Can you work these out from the model? Positions are in its coordinate system, mm. Face numbers are marked on the shaded views. Coordinates: 2 decimals unless noted, no trailing zeros. Loops run counter-clockwise (first coordinate to the right, second up) from the corner with the lowest first, then second, coordinate; pieces in that order, holes last.
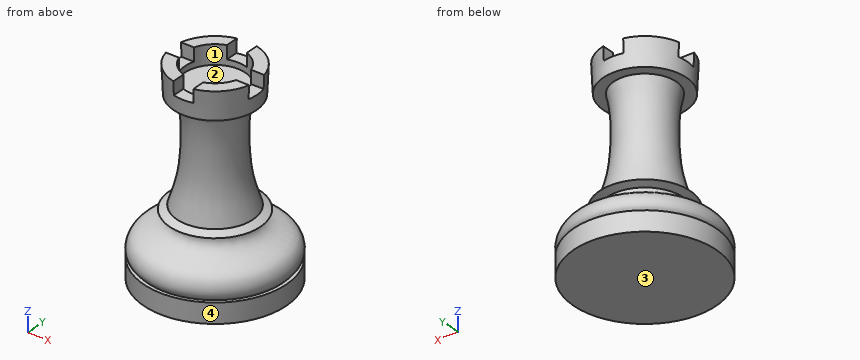
```python
from build123d import *

# Parameters (mm, degrees)
F2_W     = 2.54
F2_H     = 2.54
F3_DEPTH = 1.7018
F4_R     = 3.8696767193
F5_DEPTH = 25.4
F6_DEPTH = 0.762


with BuildPart() as f1:
    # F0 (on Front) → F1 (revolve)
    with BuildSketch(Plane.XZ):
        Polygon((0, 2.54), (0, 0), (9.1186, 0), (9.1186, 2.54), (8.6556235328, 2.54), align=None)
        with BuildLine():
            Line((0, 8.6968354881), (0, 2.54))
            Line((0, 2.54), (8.6556235328, 2.54))
            add(Edge.make_bspline(
                [(8.6556235328, 2.54), (8.8550384762, 2.7402463297), (9.3618805952, 3.2434009078), (8.6917500556, 5.5027157982), (5.7913825103, 5.9282046951), (4.8176161945, 7.0821708068), (4.8696040176, 7.7928476967)],
                knots=[0, 0, 0, 0, 0.1745078988, 0.4312211664, 0.7434636272, 1, 1, 1, 1], degree=3))
            Line((4.8696040176, 7.7928476967), (5.8183851652, 8.18317011))
            Line((5.8183851652, 8.18317011), (4.8696040176, 8.6968354881))
            Line((4.8696040176, 8.6968354881), (0, 8.6968354881))
        make_face()
        with BuildLine():
            Line((0, 25.4), (0, 8.6968354881))
            Line((0, 8.6968354881), (4.8696040176, 8.6968354881))
            add(Edge.make_bspline(
                [(4.8696040176, 8.6968354881), (4.4544059351, 9.9683403285), (3.4997394922, 12.6262885828), (3.3990850213, 19.3145075221), (3.8213017941, 21.1251515454), (3.9858142845, 21.8313997611)],
                knots=[0, 0, 0, 0, 0.3320269683, 0.74449656, 1, 1, 1, 1], degree=3))
            Line((3.9858142845, 21.8313997611), (4.8696040176, 21.8313997611))
            Line((4.8696040176, 21.8313997611), (5.3105507867, 21.8313997611))
            Line((5.3105507867, 21.8313997611), (5.4714544566, 25.4))
            Line((5.4714544566, 25.4), (0, 25.4))
        make_face()
    revolve(axis=Axis((0, 0, 12.7), (0, 0, 1)))

    # F2 (on face) → F3 (cut)
    with BuildSketch(Plane.XY.offset(25.4)):
        with BuildLine():
            Line((-1.27, -1.27), (-1.27, 1.27))
            Line((-1.27, 1.27), (-5.3220215962, 1.27))
            ThreePointArc((-5.3220215962, 1.27), (-5.4714544566, 0), (-5.3220215962, -1.27))
            Line((-5.3220215962, -1.27), (-1.27, -1.27))
        make_face()
        with BuildLine():
            Line((5.3220215962, 1.27), (1.27, 1.27))
            Line((1.27, 1.27), (1.27, -1.27))
            Line((1.27, -1.27), (5.3220215962, -1.27))
            ThreePointArc((5.3220215962, -1.27), (5.4339678252, -0.6393805947), (5.4714544566, 0))
            ThreePointArc((5.4714544566, 0), (5.4339678252, 0.6393805947), (5.3220215962, 1.27))
        make_face()
        with BuildLine():
            Line((1.27, -5.3220215962), (1.27, -1.27))
            Line((1.27, -1.27), (-1.27, -1.27))
            Line((-1.27, -1.27), (-1.27, -5.3220215962))
            ThreePointArc((-1.27, -5.3220215962), (0, -5.4714544566), (1.27, -5.3220215962))
        make_face()
        with BuildLine():
            Line((-1.27, 1.27), (1.27, 1.27))
            Line((1.27, 1.27), (1.27, 5.3220215962))
            ThreePointArc((1.27, 5.3220215962), (0, 5.4714544566), (-1.27, 5.3220215962))
            Line((-1.27, 5.3220215962), (-1.27, 1.27))
        make_face()
        Rectangle(F2_W, F2_H)
    extrude(amount=-F3_DEPTH, mode=Mode.SUBTRACT)

    # F4 (on face) → F5 (cut)
    with BuildSketch(Plane.XY.offset(23.6982)):
        Circle(F4_R)
    extrude(amount=F5_DEPTH, mode=Mode.SUBTRACT)

    # F4 (on face) → F6 (cut)
    with BuildSketch(Plane.XY.offset(23.6982)):
        Circle(F4_R)
    extrude(amount=-F6_DEPTH, mode=Mode.SUBTRACT)


solid = f1.part
```
Item 1: I need wall thicknesses on line 1 along X through (y, z) = (0, 23.6); line 2 along Z through (x, y) = (-6.5, 6). Which ranges of each line are inside material? Lowest first, please.
Results are:
line 1: x = -5.39 to -3.87, 3.87 to 5.39
line 2: z = 0 to 2.54, 2.74 to 4.52
Item 2: We'd pull the mould along Y, two halves only. Please class the marked faces 1, 2, 3 and 4: +Y half, -Y half, draft (parallel to the pull), parting line (faces both ways), or undercut.
Results are:
face 1: undercut
face 2: undercut
face 3: draft
face 4: parting line
Item 3: Suppose I cut it at A-A, the plane z = 23.25. Please give me the cut outline in (x, y), plus the area to 3 significant figures.
Results are:
outline: circle Ø10.75 at (0, 0); hole circle Ø7.74 at (0, 0)
area: 43.7 mm2
Item 4: I'm going to push flat-ended pins straight in: P1, Ø1.8, axis at y = 4, z = 24.5, coming from the -X side; P2, Ø1.8, axis at x = -4.5, z = 24, coming from the -Y side; P3, Ø1.5, axis at x = -3, z = 7, coming from the -Y side. Where does each tip first touch, or does it pass through?
Results are:
P1: stops at x = -4.46
P2: stops at y = -4.04
P3: stops at y = -5.07
